The listing builds one solid part. Answer for the finished solid, in the listing's coordinates (mm). Coordinates: 2 decimals unless noted, no trailing zeros. Loops run counter-clockwise (first coordinate to the right, second up) from the corner with the lowest first, then second, coordinate; pieces in that order, holes last. Notation, with made-up numbers: M -13.5,58.25 L -2.5,58.25 A10 ccw -2.5,64.25 Z; hole C 76.25,-32 d3. An arc over 180 degrees is marked long. Answer as a JSON object with one key per item and string values. Group by question number.
1. Straight lines are drawn through the part: L1, parallel to X at y = 3, z = 0.85; L2, parallel to Y at x = 9, z = 0.45. For each, find the intervals that lie inside material, in ascending order.
2. A cutting plane is placed at A-A on x = 54. Give the vertices of the cut face in (y, z).
3. A cutting plane is placed at B-B on y = 3. Give the vertices of the cut face in (x, z), and give its area (3 significant figures).
4. Given pin 1 (3.5 mm diameter, centred on x = 54, y = 3, fed in from -Z), flat-ended and moving along its own axis, determine where the tip first touches the part or whether it passes through.
Autodesk Inventor part; units mm, degrees
ref_plane "YZ Plane" through (0, 0, 0) normal (1, 0, 0) x (0, 1, 0)
ref_plane "XZ Plane" through (0, 0, 0) normal (0, 1, 0) x (-1, 0, 0)
ref_plane "XY Plane" through (0, 0, 0) normal (0, 0, 1) x (1, 0, 0)
sketch "Sketch1" plane through (0, 0, 0) normal (0, 0, 1) x (1, 0, 0)
  line L0 (0, 0) -> (63, 0)
  line L1 (63, 0) -> (63, 48)
  line L2 (63, 48) -> (0, 48)
  line L3 (0, 48) -> (0, 0)
  line L4 (9, 45) -> (54, 45) construction
  line L5 (54, 45) -> (54, 3) construction
  line L6 (54, 3) -> (9, 3) construction
  line L7 (9, 3) -> (9, 45) construction
  dimension "d0" = 63
  dimension "d1" = 48
  dimension "d2" = 45
  dimension "d3" = 42
  dimension "d4" = 3
  dimension "d5" = 9
  dimension "d6" = 9
  dimension "d7" = 3
extrude "Extrusion1" add sketch "Sketch1" along normal blind 1.8
hole "Hole1" at (9, 45, 0) at (54, 45, 0) at (9, 3, 0) at (54, 3, 0) direction (0, 0, 1) diameter 3.1 end through all
properties part number "Mechanical Driver Board"
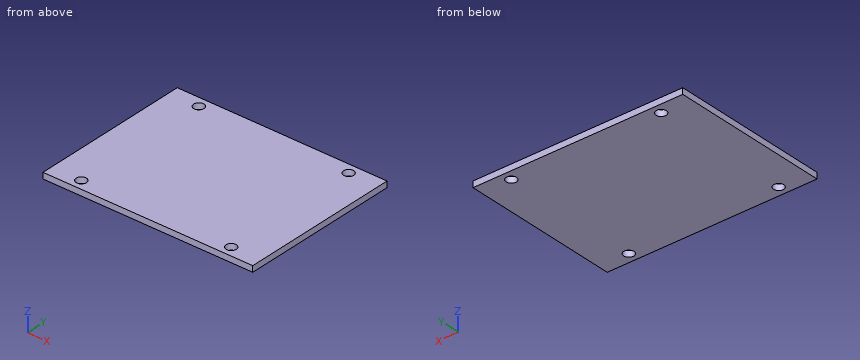
From the geometry:
{
 "1": {"L1": "x = 0 to 7.45, 10.55 to 52.45, 55.55 to 63", "L2": "y = 0 to 1.45, 4.55 to 43.45, 46.55 to 48"},
 "2": {"outline": "M 0,0 L 1.45,0 L 1.45,1.8 L 0,1.8 Z; M 4.55,0 L 43.45,0 L 43.45,1.8 L 4.55,1.8 Z; M 46.55,0 L 48,0 L 48,1.8 L 46.55,1.8 Z"},
 "3": {"outline": "M 0,0 L 7.45,0 L 7.45,1.8 L 0,1.8 Z; M 10.55,0 L 52.45,0 L 52.45,1.8 L 10.55,1.8 Z; M 55.55,0 L 63,0 L 63,1.8 L 55.55,1.8 Z", "area": "102 mm²"},
 "4": {"pin 1": "stops at z = 0"}
}
